```python
from build123d import *

# Parameters (mm, degrees)
SKETCH1_R           = 50
BOSS_EXTRUDE1_DEPTH = 200
SKETCH2_W           = 2
SKETCH2_H           = 20.463168159
BOSS_EXTRUDE2_DEPTH = 5
SKETCH3_R           = 2.5
CUT_EXTRUDE1_DEPTH  = 17
BOSS_EXTRUDE3_START = 200
SKETCH4_W           = 2
SKETCH4_H           = 10
BOSS_EXTRUDE3_DEPTH = 20.46
SKETCH5_R           = 2.5
CUT_EXTRUDE2_DEPTH  = 12.5


with BuildPart() as part:
    # Sketch1 → Boss-Extrude1 (new body)
    with BuildSketch(Plane.XY):
        Circle(SKETCH1_R)
    extrude(amount=BOSS_EXTRUDE1_DEPTH)

    # Sketch2 → Boss-Extrude2 (add, symmetric)
    with BuildSketch(Plane(origin=(0, 0, 0), x_dir=(1, 0, 0), z_dir=(0, 1, 0))):
        with Locations((-11, -210.23158408)):
            Rectangle(SKETCH2_W, SKETCH2_H)
        with Locations((11, -210.23158408)):
            Rectangle(SKETCH2_W, SKETCH2_H)
    extrude(amount=BOSS_EXTRUDE2_DEPTH, both=True)

    # Sketch3 → Cut-Extrude1 (cut, symmetric)
    with BuildSketch(Plane(origin=(0, 0, 0), x_dir=(0, 0, -1), z_dir=(1, 0, 0))):
        with Locations((-215, 0)):
            Circle(SKETCH3_R)
    extrude(amount=CUT_EXTRUDE1_DEPTH, both=True, mode=Mode.SUBTRACT)

    # Sketch4 → Boss-Extrude3 (add)
    with BuildSketch(Plane.XY.offset(BOSS_EXTRUDE3_START)):
        with Locations((-9, 0)):
            Rectangle(SKETCH4_W, SKETCH4_H)
        with Locations((9, 0)):
            Rectangle(SKETCH4_W, SKETCH4_H)
    extrude(amount=BOSS_EXTRUDE3_DEPTH)

    # Sketch5 → Cut-Extrude2 (cut, symmetric)
    with BuildSketch(Plane(origin=(0, 0, 0), x_dir=(0, 0, -1), z_dir=(1, 0, 0))):
        with Locations((-215, 0)):
            Circle(SKETCH5_R)
    extrude(amount=CUT_EXTRUDE2_DEPTH, both=True, mode=Mode.SUBTRACT)


solid = part.part
```
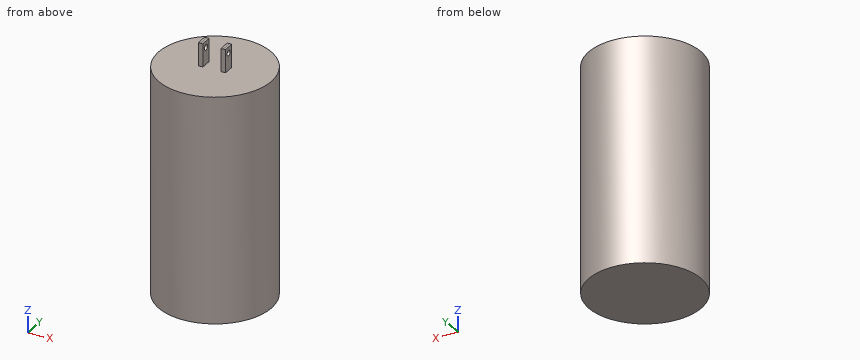
Design review of the part built by this model. Coordinates are the model's own, in mm. Coordinates: 2 decimals unless noted, no trailing zeros. Order: outer loops, then holes, each group sorted by start corner. A loop starts at its lowest first (then second) coordinate and runs counter-clockwise, first axis right, second up. Notation, with made-up numbers: (-30, 80) -> (29, 80) arc R13 cw to (29, 98) -> close; hole circle Ø2 at (24.5, 3). An arc over 180 degrees is marked (long way). One line per item, written item: value. Start each with the question number.
Q1. Take a section at D-D, the plane z = 99. State the section outline as (x, y) points, then the cut area to 3 significant figures.
Q2. Take a section at B-B, the plane y = 0. Give the number of separate pieces and of enclosed holes in the cut face, then the cut area to 3 significant figures.
Q3. Take a section at A-A, the plane z = 215. State the section outline as (x, y) points, then the cut area to 3 significant figures.
Q4. For probe 1 along Y at (x, z) = (-10.6, 215); probe 2 along Y at (x, z) = (0, 115.5); probe 3 along Z at (x, y) = (-29.5, -25), list the stretches that pass through material, from the lowest coordinate up.
Q5. Insertion check: pin 1 Ø3 at (x, y) = (26, -26.5) entering from +Z; pin 2 Ø1 at (x, y) = (9, -1) entering from +Z; pin 3 Ø5 at (y, z) = (-1.5, 212) entering from +X; pin 4 Ø4.5 at (y, z) = (0, 215) entering from -X. Each pin has a flat end and moves straight along its axis. Give the tip position at first contact, or say it passes through.
Q6. Take a section at C-C, the plane x = 0. State the section outline as (y, z) points, then the cut area to 3 significant figures.
Values follow:
1. outline: circle Ø100 at (0, 0)
1. area: 7,850 mm2
2. separate pieces: 3
2. enclosed holes: 0
2. area: 20,100 mm2
3. outline: (-12, -5) -> (-8, -5) -> (-8, -2.5) -> (-12, -2.5) -> close; (-12, 2.5) -> (-8, 2.5) -> (-8, 5) -> (-12, 5) -> close; (8, -5) -> (12, -5) -> (12, -2.5) -> (8, -2.5) -> close; (8, 2.5) -> (12, 2.5) -> (12, 5) -> (8, 5) -> close
3. area: 40.0 mm2
4. probe 1: y = -5 to -2.5, 2.5 to 5
4. probe 2: y = -50 to 50
4. probe 3: z = 0 to 200
5. pin 1: stops at z = 200
5. pin 2: stops at z = 220.46
5. pin 3: stops at x = 12
5. pin 4: passes through
6. outline: (-50, 0) -> (50, 0) -> (50, 200) -> (-50, 200) -> close
6. area: 20,000 mm2
